```python
from build123d import *

# Parameters (mm, degrees)
ESQUISSE1_R        = 1.9
ESQUISSE1_R_2      = 1.950000027
BOSS_EXTRU_1_DEPTH = 5


with BuildPart() as part:
    # Esquisse1 → Boss.-Extru.1 (new body)
    with BuildSketch(Plane.XY):
        with BuildLine():
            Line((-36.042079519, 6.612329971), (-2.756888739, -40.60806749))
            ThreePointArc((-2.756888739, -40.60806749), (-0.971927818, -42.166026475), (1.329860158, -42.727358644))
            Line((1.329860158, -42.727358644), (16.414744778, -42.727358644))
            ThreePointArc((16.414744778, -42.727358644), (18.537962215, -42.254161899), (20.25929982, -40.92413773))
            Line((20.25929982, -40.92413773), (30.250474641, -28.908411747))
            Line((30.250474641, -28.908411747), (30.250474641, -23.914585762))
            Line((30.250474641, -23.914585762), (40.110474641, -23.914585762))
            Line((40.110474641, -23.914585762), (40.110474641, 22.085414238))
            Line((40.110474641, 22.085414238), (30.250474641, 22.085414238))
            Line((30.250474641, 22.085414238), (30.289127967, 26.563728114))
            Line((30.289127967, 26.563728114), (-9.322024272, 41.369413347))
            ThreePointArc((-9.322024272, 41.369413347), (-35.395503084, 33.764537489), (-36.042079519, 6.612329971))
        make_face()
        with Locations((-29.585096552, 28.740581162)):
            Circle(ESQUISSE1_R, mode=Mode.SUBTRACT)
        with Locations((-21.4008614, 34.486736198)):
            Circle(ESQUISSE1_R, mode=Mode.SUBTRACT)
        with Locations((-1.428936876, -11.362171084)):
            Circle(ESQUISSE1_R_2, mode=Mode.SUBTRACT)
        with Locations((6.755298276, -5.616016048)):
            Circle(ESQUISSE1_R_2, mode=Mode.SUBTRACT)
        with Locations((10.104149324, 21.053484932)):
            Circle(ESQUISSE1_R, mode=Mode.SUBTRACT)
        with Locations((3.608581782, -37.743606202)):
            Circle(ESQUISSE1_R, mode=Mode.SUBTRACT)
        with Locations((13.608573866, -37.73091599)):
            Circle(ESQUISSE1_R, mode=Mode.SUBTRACT)
        with Locations((35.110474641, -17.914585762)):
            Circle(ESQUISSE1_R, mode=Mode.SUBTRACT)
        with Locations((35.110474641, 16.085214419)):
            Circle(ESQUISSE1_R, mode=Mode.SUBTRACT)
        with BuildLine():
            Line((-14.809164556, 33.799672662), (-20.660891689, 29.691172522))
            ThreePointArc((-20.660891689, 29.691172522), (-22.18628804, 29.363713126), (-23.482781796, 30.231565432))
            Line((-23.482781796, 30.231565432), (-25.924897053, 33.709865414))
            ThreePointArc((-25.924897053, 33.709865414), (-26.47826462, 34.0839702), (-27.131559209, 33.944771651))
            ThreePointArc((-27.131559209, 33.944771651), (-27.478774003, 33.409530528), (-27.357701898, 32.783125931))
            Line((-27.357701898, 32.783125931), (-24.915585604, 29.304825893))
            ThreePointArc((-24.915585604, 29.304825893), (-24.495010021, 27.771470128), (-25.32590655, 26.415861527))
            Line((-25.32590655, 26.415861527), (-31.177633683, 22.307361387))
            Line((-31.177633683, 22.307361387), (-8.020629273, -10.675105791))
            Line((-8.020629273, -10.675105791), (-2.16890246, -6.566605875))
            ThreePointArc((-2.16890246, -6.566605875), (-0.674874752, -6.233398064), (0.617175813, -7.054221782))
            Line((0.617175813, -7.054221782), (3.05929141, -10.532521451))
            ThreePointArc((3.05929141, -10.532521451), (3.608413847, -10.881372123), (4.243376724, -10.739758611))
            ThreePointArc((4.243376724, -10.739758611), (4.592227421, -10.190636157), (4.450613892, -9.555673255))
            Line((4.450613892, -9.555673255), (2.008497767, -6.077373005))
            ThreePointArc((2.008497767, -6.077373005), (1.675290093, -4.583345549), (2.496113536, -3.291295137))
            Line((2.496113536, -3.291295137), (8.347839718, 0.817205678))
            Line((8.347839718, 0.817205678), (-14.809164556, 33.799672662))
        make_face(mode=Mode.SUBTRACT)
    extrude(amount=BOSS_EXTRU_1_DEPTH)


solid = part.part
```
Design review of the part built by this model. Coordinates are the model's own, in mm. A direction names the side the tool comes from. Coordinates: 2 decimals unless noted, no trailing zeros. Order: outer loops, then holes, each group sorted by start corner. A loop starts at its lowest first (then second) coordinate and runs counter-clockwise, first axis right, second up.
1) Take a section at B-B, the plane y = 12. Give the boundary of the cut face in (x, z), and give its area (3 significant figures).
2) Take a section at C-C, the plane x = 7. Give the boundary of the cut face in (y, z), and give its area (3 significant figures).
3) Take a section at D-D, the plane z = 2. State how many separate pieces and enclosed holes the cut face has, and give its area (3 significant figures).
4) Take a section at A-A, the plane x = -17. Give the boundary of the cut face in (y, z), and give its area (3 significant figures).
5) Mouldability with a two-part tool opening along Y and no side actions: class faces 4 (the cylindrical face through (-1.68, -9.43, 2.46)), 5 (the flat face through (35, -23.915, 2)), 6 (the flat face through (40.11, -1, 2)) as +Y half, -Y half, draft (parallel to the pull), parting line (faces both ways), or undercut.
6) Wall thickness on line 1 along Y through (x, z) = (-29.5, 4.4); line 2 along Y through (x, z) = (36, 1.4); line 3 along X through (y, z) = (-4.5, 1.75): over which ranges is each line inside the solid? List them lowest first.
7) For faces 1 (the flat face through (-19.761, 6.047, 2.465)), 2 (the flat face through (-19.63, -16.67, 2.46)), 3 (the flat face through (30.25, -26, 2)), list the 3-axis set-ups (+Z, -Z, +X, -X, +Y, -Y) from which the entire face can be reached by the end or side of a thin tool; tool diameter is ignored.
8) Clearance check with flat-ended pins moving along their axes: pin 1 (3 mm diameter, centred on y = 33, z = 2, fed in from -X); pin 2 (1.5 mm diameter, centred on y = -27, z = 4, fed in from +X); pin 3 (3 mm diameter, centred on y = 13.5, z = 3, fed in from -X). State where each tip first meets the part, or that it passes through.
Returned:
1. outline: (-38.82, 0) - (-23.94, 0) - (-23.94, 5) - (-38.82, 5) - close; (0.5, 0) - (40.11, 0) - (40.11, 5) - (0.5, 5) - close
1. area: 272 mm2
2. outline: (-42.73, 0) - (-7.55, 0) - (-7.55, 5) - (-42.73, 5) - close; (-3.68, 0) - (-0.13, 0) - (-0.13, 5) - (-3.68, 5) - close; (2.74, 0) - (35.27, 0) - (35.27, 5) - (2.74, 5) - close
2. area: 356 mm2
3. separate pieces: 1
3. enclosed holes: 10
3. area: 3,910 mm2
4. outline: (-20.4, 0) - (2.11, 0) - (2.11, 5) - (-20.4, 5) - close; (32.26, 0) - (42.75, 0) - (42.75, 5) - (32.26, 5) - close
4. area: 165 mm2
5. face 4: undercut
5. face 5: -Y half
5. face 6: draft
6. line 1: y = -2.67 to 19.92, 23.49 to 26.84, 30.64 to 39.16
6. line 2: y = -23.91 to -19.59, -16.24 to 14.41, 17.76 to 22.09
6. line 3: x = -28.21 to -12.36, 1.69 to 5.16, 8.35 to 40.11
7. face 1: +Z, -Z
7. face 2: +Z, -Z, -X, -Y
7. face 3: +Z, -Z, +X, -Y
8. pin 1: stops at x = -36.93
8. pin 2: stops at x = 30.25
8. pin 3: stops at x = -39.67
